Check sheet for the modelled part. Datum: model origin and axes. Units: mm. Give positions to 0.01 mm unless a question says otherwise; leave off trailing zeros. Loops run counter-clockwise (first coordinate to the right, second up) from the corner with the lowest first, then second, coordinate; pieces in that order, holes last. Notation, with made-up numbers: (-13, 81) - (0, 81) arc R24 cw to (0, 105) - close; hole circle Ø10 at (47.25, -16.75). An arc over 180 degrees is marked (long way). Use one line per item in the form item = value.
from build123d import *

# Parameters (mm, degrees)
SKETCH1_W                 = 88.9
SKETCH1_H                 = 84.12226
BOSS_EXTRUDE1_DEPTH       = 2.54
SKETCH2_R                 = 5.08
CUT_EXTRUDE1_DEPTH        = 2.54
SKETCH3_R                 = 12.065
CUT_EXTRUDE2_DEPTH        = 74.692319271
SKETCH4_R                 = 0.889
SKETCH4_W                 = 23.876
SKETCH4_H                 = 11.7094
CUT_EXTRUDE3_DEPTH        = 74.692319271
F_6_CLEARANCE_HOLE1_D     = 3.7973
BOSS_EXTRUDE2_DEPTH       = 2.54
SKETCH10_W                = 2.54
SKETCH10_H                = 12.446
CUT_EXTRUDE4_DEPTH        = 172.20227832
LPATTERN1_COUNT           = 4
LPATTERN1_PITCH           = 25.4
SKETCH11_W                = 25.4
SKETCH11_H                = 2.54
BOSS_EXTRUDE3_DEPTH       = 2.54
LPATTERN2_COUNT           = 4
LPATTERN2_PITCH           = 50.8
LPATTERN2_COUNT_DIR2      = 2
LPATTERN2_PITCH_DIR2      = 152.654
SKETCH12_W                = 2.54
SKETCH12_H                = 25.019
BOSS_EXTRUDE4_DEPTH       = 2.54
LPATTERN3_COUNT           = 3
LPATTERN3_PITCH           = 50.038
SKETCH13_W                = 13.02766
SKETCH13_H                = 155.194
CUT_EXTRUDE5_DEPTH        = 175.774762566
F_6_CLEARANCE_HOLE2_D     = 3.6576
SKETCH17_W                = 12.7
SKETCH17_H                = 155.194
BOSS_EXTRUDE5_DEPTH       = 2.54
LPATTERN4_COUNT           = 2
LPATTERN4_PITCH           = 192.71234
LPATTERN4_COPY_1_SKETCH_W = 2.54
LPATTERN4_COPY_1_SKETCH_H = 25.019
LPATTERN4_COPY_1_DEPTH    = 2.54
LPATTERN4_COPY_2_SKETCH_W = 2.54
LPATTERN4_COPY_2_SKETCH_H = 25.019
LPATTERN4_COPY_2_DEPTH    = 2.54
SKETCH18_W                = 25.4
SKETCH18_H                = 19.05
CUT_EXTRUDE6_DEPTH        = 175.774762566
FILLET1_R                 = 3.175
CUT_EXTRUDE7_DEPTH        = 2.54
LPATTERN5_COUNT           = 6
LPATTERN5_PITCH           = 7.62
F_6_CLEARANCE_HOLE3_D     = 3.6576
F_6_CLEARANCE_HOLE3_DEPTH = 9.398
F_6_CLEARANCE_HOLE3_TIP   = 1.0988539


with BuildPart() as part:
    # Sketch1 → Boss-Extrude1 (new body)
    with BuildSketch(Plane(origin=(0, 0, 0), x_dir=(1, 0, 0), z_dir=(0, 1, 0))):
        with Locations((0, -16.66113)):
            Rectangle(SKETCH1_W, SKETCH1_H)
    extrude(amount=BOSS_EXTRUDE1_DEPTH)

    # Sketch2 → Cut-Extrude1 (cut)
    with BuildSketch(Plane(origin=(0, 2.54, 0), x_dir=(1, 0, 0), z_dir=(0, 1, 0))):
        with Locations((-28.1548967, 7.85)):
            Circle(SKETCH2_R)
        with BuildLine():
            Line((-25.6148967, 15.65), (-30.6948967, 15.65))
            ThreePointArc((-30.6948967, 15.65), (-32.3948967, 17.35), (-30.6948967, 19.05))
            Line((-30.6948967, 19.05), (-25.6148967, 19.05))
            ThreePointArc((-25.6148967, 19.05), (-23.9148967, 17.35), (-25.6148967, 15.65))
        make_face()
        with BuildLine():
            Line((-30.6948967, 0.05), (-25.6148967, 0.05))
            ThreePointArc((-25.6148967, 0.05), (-23.9148967, -1.65), (-25.6148967, -3.35))
            Line((-25.6148967, -3.35), (-30.6948967, -3.35))
            ThreePointArc((-30.6948967, -3.35), (-32.3948967, -1.65), (-30.6948967, 0.05))
        make_face()
        with BuildLine():
            Line((-37.6798967, 9.55), (-18.6298967, 9.55))
            ThreePointArc((-18.6298967, 9.55), (-16.9298967, 7.85), (-18.6298967, 6.15))
            Line((-18.6298967, 6.15), (-37.6798967, 6.15))
            ThreePointArc((-37.6798967, 6.15), (-39.3798967, 7.85), (-37.6798967, 9.55))
        make_face()
    cut_extrude1 = extrude(amount=-CUT_EXTRUDE1_DEPTH, mode=Mode.SUBTRACT)

    # Mirror1: Cut-Extrude1 across plane
    add(cut_extrude1.mirror(Plane(origin=(0, 0, 0), x_dir=(0, 0, 1), z_dir=(1, 0, 0))), mode=Mode.SUBTRACT)

    # Sketch3 → Cut-Extrude2 (cut, through all)
    with BuildSketch(Plane(origin=(0, 2.54, 0), x_dir=(1, 0, 0), z_dir=(0, 1, 0))):
        with Locations(Location((0, -32.6884, 0), (0, 0, 270))):
            Circle(SKETCH3_R)
    extrude(amount=-CUT_EXTRUDE2_DEPTH, mode=Mode.SUBTRACT)

    # Sketch4 → Cut-Extrude3 (cut, through all)
    with BuildSketch(Plane(origin=(0, 2.54, 0), x_dir=(1, 0, 0), z_dir=(0, 1, 0))):
        with Locations(Location((-20.0787, -52.86756, 0), (0, 0, 270))):
            Circle(SKETCH4_R)
        with Locations(Location((8.2423, -52.86756, 0), (0, 0, 270))):
            Circle(SKETCH4_R)
        with Locations((-5.9182, -52.86756)):
            Rectangle(SKETCH4_W, SKETCH4_H)
    extrude(amount=-CUT_EXTRUDE3_DEPTH, mode=Mode.SUBTRACT)

    # #6 Clearance Hole1 (through all)
    with Locations(Plane(origin=(0, 2.54, 0), x_dir=(1, 0, 0), z_dir=(0, 1, 0))):
        with Locations((0, 1.4986), (-8.128, -13.7414), (8.128, -13.7414)):
            Hole(F_6_CLEARANCE_HOLE1_D / 2)

    # Sketch9 → Boss-Extrude2 (add)
    with BuildSketch(Plane(origin=(0, 0, 0), x_dir=(1, 0, 0), z_dir=(0, 1, 0))):
        Polygon((-44.45, 25.4), (44.45, 25.4), (44.45, -58.72226), (6.0198, -58.72226), (6.0198, -59.23026), (-17.8562, -59.23026), (-17.8562, -58.72226), (-44.45, -58.72226), (-44.45, -107.74426), (133.02234, -107.74426), (133.02234, 42.36974), (-44.45, 42.36974), align=None)
    extrude(amount=BOSS_EXTRUDE2_DEPTH)

    # Sketch10 → Cut-Extrude4 (cut, through all)
    with BuildSketch(Plane(origin=(0, 2.54, 0), x_dir=(1, 0, 0), z_dir=(0, 1, 0))):
        with Locations((97.03054, 5.41274)):
            Rectangle(SKETCH10_W, SKETCH10_H)
    cut_extrude4 = extrude(amount=-CUT_EXTRUDE4_DEPTH, mode=Mode.SUBTRACT)

    # LPattern1: Cut-Extrude4 ×4
    with Locations(*[(0, 0, i * LPATTERN1_PITCH) for i in range(1, LPATTERN1_COUNT)]):
        add(cut_extrude4, mode=Mode.SUBTRACT)

    # Sketch11 → Boss-Extrude3 (add)
    with BuildSketch(Plane(origin=(0, 2.54, 0), x_dir=(1, 0, 0), z_dir=(0, 1, 0))):
        with Locations((107.62234, -109.01426)):
            Rectangle(SKETCH11_W, SKETCH11_H)
    boss_extrude3 = extrude(amount=-BOSS_EXTRUDE3_DEPTH)

    # LPattern2: Boss-Extrude3 4 × 2
    with Locations(*[(-i * LPATTERN2_PITCH, 0, -j * LPATTERN2_PITCH_DIR2) for i in range(LPATTERN2_COUNT) for j in range(LPATTERN2_COUNT_DIR2) if (i, j) != (0, 0)]):
        add(boss_extrude3)

    # Sketch12 → Boss-Extrude4 (add)
    with BuildSketch(Plane(origin=(0, 2.54, 0), x_dir=(1, 0, 0), z_dir=(0, 1, 0))):
        with Locations((134.29234, -82.72526)):
            Rectangle(SKETCH12_W, SKETCH12_H)
    boss_extrude4 = extrude(amount=-BOSS_EXTRUDE4_DEPTH)

    # LPattern3: Boss-Extrude4 ×3
    with Locations(*[(0, 0, -i * LPATTERN3_PITCH) for i in range(1, LPATTERN3_COUNT)]):
        add(boss_extrude4)

    # Sketch13 → Cut-Extrude5 (cut, through all)
    with BuildSketch(Plane(origin=(0, 2.54, 0), x_dir=(1, 0, 0), z_dir=(0, 1, 0))):
        with Locations((-50.96383, -32.68726)):
            Rectangle(SKETCH13_W, SKETCH13_H)
    extrude(amount=-CUT_EXTRUDE5_DEPTH, mode=Mode.SUBTRACT)

    # #6 Clearance Hole2 (through all)
    with Locations(Plane(origin=(0, 0, 0), x_dir=(-1, 0, 0), z_dir=(0, -1, 0))):
        with Locations((6.990100066, 31.390026268), (-6.979899934, 31.390026268)):
            Hole(F_6_CLEARANCE_HOLE2_D / 2)

    # Sketch17 → Boss-Extrude5 (add)
    with BuildSketch(Plane(origin=(0, 2.54, 0), x_dir=(1, 0, 0), z_dir=(0, 1, 0))):
        with Locations((-50.8, -32.68726)):
            Rectangle(SKETCH17_W, SKETCH17_H)
    extrude(amount=-BOSS_EXTRUDE5_DEPTH)

    # LPattern4: Boss-Extrude4 ×2
    with Locations(*[(-i * LPATTERN4_PITCH, 0, 0) for i in range(1, LPATTERN4_COUNT)]):
        add(boss_extrude4)

    # LPattern4 copy 1 sketch → LPattern4 copy 1 (add)
    with BuildSketch(Plane(origin=(-192.71234, 2.54, -50.038), x_dir=(1, 0, 0), z_dir=(0, 1, 0))):
        with Locations((134.29234, -82.72526)):
            Rectangle(LPATTERN4_COPY_1_SKETCH_W, LPATTERN4_COPY_1_SKETCH_H)
    extrude(amount=-LPATTERN4_COPY_1_DEPTH)

    # LPattern4 copy 2 sketch → LPattern4 copy 2 (add)
    with BuildSketch(Plane(origin=(-192.71234, 2.54, -100.076), x_dir=(1, 0, 0), z_dir=(0, 1, 0))):
        with Locations((134.29234, -82.72526)):
            Rectangle(LPATTERN4_COPY_2_SKETCH_W, LPATTERN4_COPY_2_SKETCH_H)
    extrude(amount=-LPATTERN4_COPY_2_DEPTH)

    # Sketch18 → Cut-Extrude6 (cut, through all)
    with BuildSketch(Plane(origin=(0, 2.54, 0), x_dir=(1, 0, 0), z_dir=(0, 1, 0))):
        with Locations((38.1, -22.225)):
            Rectangle(SKETCH18_W, SKETCH18_H)
    extrude(amount=-CUT_EXTRUDE6_DEPTH, mode=Mode.SUBTRACT)

    # Fillet1
    fillet1_edges = [part.edges().sort_by_distance(p)[0] for p in [
        (25.4, 1.27, 31.75),
        (25.4, 1.27, 12.7),
        (50.8, 1.27, 12.7),
        (50.8, 1.27, 31.75),
    ]]
    fillet(fillet1_edges, radius=FILLET1_R)

    # Sketch19 → Cut-Extrude7 (cut)
    with BuildSketch(Plane(origin=(0, 2.54, 0), x_dir=(1, 0, 0), z_dir=(0, 1, 0))):
        with BuildLine():
            Line((34.29, -46.0375), (34.29, -55.5625))
            ThreePointArc((34.29, -55.5625), (33.02, -56.8325), (31.75, -55.5625))
            Line((31.75, -55.5625), (31.75, -46.0375))
            ThreePointArc((31.75, -46.0375), (33.02, -44.7675), (34.29, -46.0375))
        make_face()
    cut_extrude7 = extrude(amount=-CUT_EXTRUDE7_DEPTH, mode=Mode.SUBTRACT)

    # LPattern5: Cut-Extrude7 ×6, 2 skipped
    with Locations(*[(i * LPATTERN5_PITCH, 0, 0) for i in range(1, LPATTERN5_COUNT) if i not in (1, 4)]):
        add(cut_extrude7, mode=Mode.SUBTRACT)

    # #6 Clearance Hole3
    with Locations(Plane(origin=(0, 2.54, 0), x_dir=(1, 0, 0), z_dir=(0, 1, 0))):
        with Locations((-47.625, 35.38474), (-47.625, -100.75926), (123.49734, -100.75926), (123.49734, 35.38474)):
            Hole(F_6_CLEARANCE_HOLE3_D / 2, depth=F_6_CLEARANCE_HOLE3_DEPTH)
            with Locations((0, 0, -(F_6_CLEARANCE_HOLE3_DEPTH + F_6_CLEARANCE_HOLE3_TIP / 2))):  # 118° drill point
                Cone(0, F_6_CLEARANCE_HOLE3_D / 2, F_6_CLEARANCE_HOLE3_TIP, mode=Mode.SUBTRACT)


solid = part.part
Item 1: Thickness scan on L1, parallel to Z at x = 21.5, y = 0.85; L2, parallel to X at y = 1.8, z = -12.5; L3, parallel to X at y = 2, z = 2. Record the ranges inside material, lowest first.
Answer block:
L1 = -42.37 to -9.55, -6.15 to 107.74
L2 = -59.69 to -30.2, -26.11 to 26.11, 30.2 to 135.56
L3 = -57.15 to -32.36, -23.95 to 23.95, 32.36 to 133.02
Item 2: Mould release check, pull along X, two halves, no side actions. Record for faces 1 (the face through (37, 0, 49)), 2 (the face through (0.25, 1.25, -3.38)): released by +X, released by -X, zero draft, split by the parting line, or undercut.
Answer block:
face_1 = zero draft
face_2 = undercut
Item 3: Gauge pin test, flat ends, axial feed: P1, Ø0.8, axis at y = 1.5, z = 109.5, coming from the +X side; P2, Ø1.3, axis at x = -20.5, y = 1, coming from the -Z side. Record the tip position at first contact, or that the pin passes through.
Answer block:
P1 = 120.32
P2 = -42.37
Item 4: Section check B-B on y = 2.1. Give the number of separate pieces and of enclosed holes in the cut face, then the cut area to 3 significant figures.
Answer block:
separate_pieces = 1
enclosed_holes = 28
area = 27,500 mm2
Item 5: Section check A-A on x = 77. Record the boundary of the cut face in (y, z).
Answer block:
outline = (0, -42.37) - (2.54, -42.37) - (2.54, 107.74) - (0, 107.74) - close
